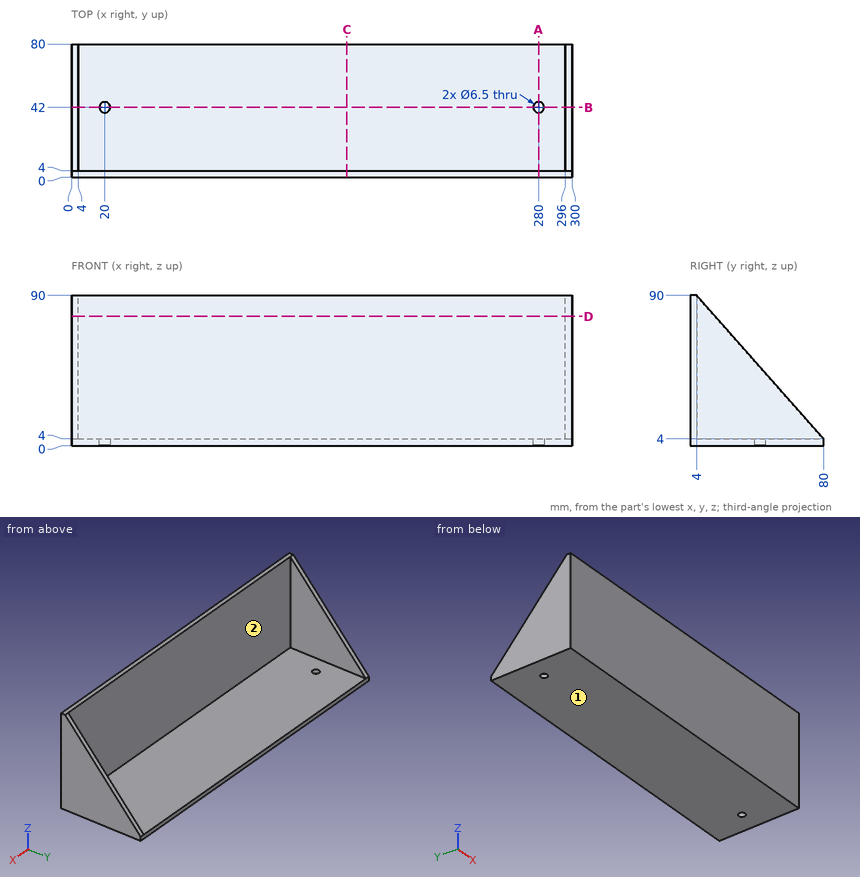
Input: dimensioned drawing with shaded views. Units: mm. Origin: part minimum x, y, z. A direction names the side the tool comes from. Round coordinates to 2 decimals unless told otherwise and drop trailing zeros. Order: outer loops, then holes, each group sorted by start corner. A loop starts at its lowest first (then second) coordinate and runs counter-clockwise, first axis right, second up.
1. Pin query (flat end, axial travel): P1, Ø12, axis at x = 188, y = 20, coming from the +Z side; P2, Ø12, axis at x = 70.5, z = 42.5, coming from the +Y side. Return the tip coordinate at first contact, or that it passes through.
The answers:
P1: stops at z = 4
P2: stops at y = 4
2. Cut plane C-C, the plane x = 165. Output: boundary loops of the cut face in (y, z), then the cut area to 3 significant figures.
The answers:
outline: (0, 0) - (80, 0) - (80, 4) - (4, 4) - (4, 90) - (0, 90) - close
area: 664 mm2
3. Material intervals for line 1 (Y direction, x = 280, z = 1.3); line 2 (X direction, y = 8, z = 80); line 3 (Z direction, x = 35, y = 62), sorted ascending.
The answers:
line 1: y = 0 to 38.75, 45.25 to 80
line 2: x = 0 to 4, 296 to 300
line 3: z = 0 to 4
4. Cut plane D-D, the plane z = 77.5. Output: boundary loops of the cut face in (x, y).
The answers:
outline: (0, 0) - (300, 0) - (300, 15.05) - (296, 15.05) - (296, 4) - (4, 4) - (4, 15.05) - (0, 15.05) - close
5. Cut plane B-B, the plane y = 42. Output: boundary loops of the cut face in (x, z), then the cut area to 3 significant figures.
The answers:
outline: (0, 0) - (16.75, 0) - (16.75, 4) - (4, 4) - (4, 47) - (0, 47) - close; (23.25, 0) - (276.75, 0) - (276.75, 4) - (23.25, 4) - close; (283.25, 0) - (300, 0) - (300, 47) - (296, 47) - (296, 4) - (283.25, 4) - close
area: 1,490 mm2
6. Cut plane A-A, the plane x = 280. Output: boundary loops of the cut face in (y, z), then the cut area to 3 significant figures.
The answers:
outline: (0, 0) - (38.75, 0) - (38.75, 4) - (4, 4) - (4, 90) - (0, 90) - close; (45.25, 0) - (80, 0) - (80, 4) - (45.25, 4) - close
area: 638 mm2
7. Set-up query: the marked faces 1 and 2. Return all of +Z, -Z, +X, -X, +Y, -Y with unobstructed straight access to the full face (end or side cutting, diameter ignored); none if empty.
The answers:
face 1: -Z, +X, -X, +Y, -Y
face 2: +Z, +Y
